Read the model definition and answer for the solid it produces. Units are mm, in the model's axes. A direction names the side the tool comes from. Coordinates: 2 decimals unless noted, no trailing zeros. Write each loop counter-clockwise with the first axis right and the second up, starting at its lowest first coordinate (ties: lowest second). Pieces come first, ordered by that corner, then holes. Notation, with made-up numbers: (9.25, 46) -> (35.25, 46) arc R31 ccw to (35.25, 79) -> close; hole circle Ø9 at (13, 44). An arc over 180 degrees is marked (long way). Answer in a Markdown table with one row per item. Add a question column.
Item 1: Section B-B on y = -35.5 is taken. Write down the section's boundary in (x, z), then the cut area to 3 significant figures.
Item 2: Section A-A on z = 48 is taken. Write down the section's boundary in (x, y).
Item 3: Straight lines are drawn through the part: line 1 (Z direction, x = 10, y = -40); line 2 (Y direction, x = 18, z = 34.5). For each, find the intervals that lie inside material, in ascending order. Write a range as from..to.
Item 4: Section D-D on y = -10 is taken. Write down the section's boundary in (x, z), then the cut area to 3 significant figures.
Item 5: Given pin 1 Ø1.6 at (y, z) = (7.5, 41.5) entering from +X; pin 2 Ø3 at (x, y) = (12.5, -49.5) entering from +Z; pin 3 Ø20 at (y, z) = (-50, 18.5) entering from +X; pin 4 Ø1 at (y, z) = (-24.5, 22.5) entering from -X, each flat-ended and moving along its own axis, determine where each tip first touches the part or whether it passes through.
Item 6: Section C-C on z = 34 is taken. Write down the section's boundary in (x, y).
Item 7: For a pull along Y with two mould halves and no side action, classify faces 5 (the face through (8, -45, 44.852)), 6 (the face through (29, 12.038, 43)), 7 (the face through (29, 3, 40.223)), 8 (the face through (23, -33.682, 35)) as +Y half, -Y half, draft (parallel to the pull), parting line (faces both ways), or undercut.
Item 8: Which of the six approach directions +Z, -Z, +X, -X, +Y, -Y give full straight-line access (tool end or side, diameter ignored) to faces 1 (the face through (25, -31.142, 31)), 2 (the face through (8, -45, 29.717)), 3 (the face through (3.918, -33.197, 34.806)), 4 (the face through (2.54, -46, 49))?
```python
from build123d import *

# Parameters (mm, degrees)
F0_W        = 28.7528
F0_H        = 19.3099416792
F1_DEPTH    = 38.354
F2_DEPTH    = 25.146
F3_R        = 20.8491483247
F5_DEPTH    = 29.972
F6_T        = 2.54
F6_T3_DEPTH = 33.8328
F8_W        = 5.5572818965
F8_H        = 5.2297823131
F9_DEPTH    = 17.78
F9_FACE_W   = 5.5572818965
F9_FACE_H   = 5.2297823131
F7_W        = 38.354
F7_H        = 44.4559416792
F7_R        = 5.5881190885
F10_DEPTH   = 25.4


# Not quite as in the source:
# - a shell that OpenCascade refuses in one call is made with other operations: the cavity is built on its own and cut out


with BuildPart() as f1:
    # F0 (on Right) → F1 (new body)
    with BuildSketch(Plane.YZ):
        with Locations((-45.5179288597, 21.1969297379)):
            Rectangle(F0_W, F0_H)
    extrude(amount=F1_DEPTH)

    # F2 (add): a face of the model
    f2_faces = [f1.faces().sort_by_distance(p)[0] for p in [
        (19.177, -45.5179288597, 30.8519005775),
    ]]
    extrude(f2_faces, amount=F2_DEPTH)

    # F3
    f3_edges = [f1.edges().sort_by_distance(p)[0] for p in [
        (38.354, -59.894329, 33.76993),
    ]]
    fillet(f3_edges, radius=F3_R)

    # F4 (on face) → F5 (cut)
    with BuildSketch(Plane.XZ.offset(59.8943288597)):
        Polygon((5.3893399472, 32.2574861348), (11.1945441877, 32.2574861348), (14.0971463079, 37.2849404812), (11.1945441877, 42.3123948276), (5.3893399472, 42.3123948276), (2.486737827, 37.2849404812), align=None)
    extrude(amount=-F5_DEPTH, mode=Mode.SUBTRACT)

    # F6: shell of thickness 2.54, made by hand


with BuildPart() as f6_core1:
    # F6_t2: copy of F1
    add(f1.part)

    # the walls: a layer under each face that stays
    f6_faces = [f6_core1.faces().sort_by_distance(p)[0] for p in [
        (14.5873763961, -59.8943288597, 48.5885769643),
        (19.177, -45.5179288597, 11.5419588983),
        (32.2474258377, -53.7877546974, 33.7699297379),
        (0, -45.5179288597, 33.7699297379),
        (3.9380388871, -45.5179288597, 39.7986676544),
        (8.2919420674, -45.5179288597, 42.3123948276),
        (12.6458452478, -45.5179288597, 39.7986676544),
        (12.6458452478, -45.5179288597, 34.771213308),
        (8.2919420674, -45.5179288597, 32.2574861348),
        (3.9380388871, -45.5179288597, 34.771213308),
        (38.354, -35.0933546974, 33.7699297379),
        (19.177, -31.1415288597, 33.7699297379),
    ]]
    thicken(f6_faces, amount=-F6_T, mode=Mode.SUBTRACT)

    # F6_s4 → F6_t3 (cut)
    with BuildSketch(Plane.XZ.offset(28.6015288597)):
        Polygon((2.5307319175, 37.2849404812), (0.2870333013, 38.5549404812), (-0.4462015405, 37.2849404812), (0.2870333013, 36.0149404812), align=None)
        Polygon((5.4113369925, 42.2742948276), (3.1896354216, 43.5823948276), (3.9228702635, 44.8523948276), (5.3893399472, 44.8523948276), align=None)
        Polygon((11.1725471424, 42.2742948276), (11.1945441877, 44.8523948276), (12.6610138714, 44.8523948276), (13.3942487133, 43.5823948276), align=None)
        Polygon((14.0531522174, 37.2849404812), (16.2968508335, 38.5549404812), (17.0300856754, 37.2849404812), (16.2968508335, 36.0149404812), align=None)
        Polygon((11.1725471424, 32.2955861348), (13.3942487133, 30.9874861348), (12.6610138714, 29.7174861348), (11.1945441877, 29.7174861348), align=None)
        Polygon((5.4113369925, 32.2955861348), (5.3893399472, 29.7174861348), (3.9228702635, 29.7174861348), (3.1896354216, 30.9874861348), align=None)
    extrude(amount=F6_T3_DEPTH, mode=Mode.SUBTRACT)


with BuildPart() as f1_1:
    add(f1.part)

    # what is left inside the walls is the cavity
    f6_cavity = [f6_core1.part.solids().sort_by_distance(p)[0] for p in [
        (24.722667, -33.706929, 35.03993),
    ]]
    add(f6_cavity, mode=Mode.SUBTRACT)

    # F8 (on face) → F9 (join)
    with BuildSketch(Plane(origin=(0, -31.1415288597, 0), x_dir=(-1, 0, 0), z_dir=(0, 1, 0))):
        with Locations((-28.6376820877, 42.8374167532)):
            Rectangle(F8_W, F8_H)
    extrude(amount=F9_DEPTH)

    # F9_face (on face) + F7 (on face) → F10 (join)
    with BuildSketch(Plane(origin=(28.6376820877, -13.3615288597, 42.8374167532), x_dir=(-1, 0, 0), z_dir=(0, 1, 0))):
        Rectangle(F9_FACE_W, F9_FACE_H)
    with BuildSketch(Plane(origin=(0, -31.1415288597, 0), x_dir=(-1, 0, 0), z_dir=(0, 1, 0))):
        with Locations((-19.177, 33.7699297379)):
            Rectangle(F7_W, F7_H)
        with Locations((-25.0183418393, 30.7178907096)):
            Circle(F7_R, mode=Mode.SUBTRACT)
        Polygon((-5.3893399472, 42.3123948276), (-2.486737827, 37.2849404812), (-5.3893399472, 32.2574861348), (-11.1945441877, 32.2574861348), (-14.0971463079, 37.2849404812), (-11.1945441877, 42.3123948276), align=None, mode=Mode.SUBTRACT)
    extrude(amount=F10_DEPTH)


solid = f1_1.part
```
Results below:
| question | item | result |
|---|---|---|
| 1 | outline | (0, 11.54) -> (38.35, 11.54) -> (38.35, 56) -> (35.81, 56) -> (35.81, 14.08) -> (2.54, 14.08) -> (2.54, 32.11) -> (3.92, 29.72) -> (12.66, 29.72) -> (17.03, 37.28) -> (12.66, 44.85) -> (3.92, 44.85) -> (2.54, 42.46) -> (2.54, 56) -> (0, 56) -> close; hole (2.49, 37.28) -> (5.39, 32.26) -> (11.19, 32.26) -> (14.1, 37.28) -> (11.19, 42.31) -> (5.39, 42.31) -> close |
| 1 | area | 406 mm2 |
| 2 | outline | (0, -59.89) -> (17.5, -59.89) arc R20.85 ccw to (38.35, -39.05) -> (38.35, -5.74) -> (0, -5.74) -> close; hole (2.54, -57.35) -> (17.5, -57.35) arc R18.31 ccw to (35.81, -39.05) -> (35.81, -33.68) -> (2.54, -33.68) -> close |
| 3 | line 1 | z = 11.54..14.08, 29.72..32.26, 42.31..44.85 |
| 3 | line 2 | y = -59.89..-57.35, -33.68..-5.74 |
| 4 | outline | (0, 11.54) -> (38.35, 11.54) -> (38.35, 56) -> (0, 56) -> close; hole (2.49, 37.28) -> (5.39, 32.26) -> (11.19, 32.26) -> (14.1, 37.28) -> (11.19, 42.31) -> (5.39, 42.31) -> close; hole circle Ø11.18 at (25.02, 30.72) |
| 4 | area | 1,520 mm2 |
| 5 | pin 1 | stops at x = 31.42 |
| 5 | pin 2 | stops at z = 44.85 |
| 5 | pin 3 | stops at x = 38.33 |
| 5 | pin 4 | stops at x = 0 |
| 6 | outline | (0, -59.89) -> (4.38, -59.89) -> (4.38, -5.74) -> (0, -5.74) -> close; (12.2, -59.89) -> (17.5, -59.89) arc R20.85 ccw to (38.35, -39.05) -> (38.35, -5.74) -> (29.54, -5.74) -> (29.54, -31.14) -> (20.5, -31.14) -> (20.5, -5.74) -> (12.2, -5.74) -> close; hole (15.13, -57.35) -> (17.5, -57.35) arc R18.31 ccw to (35.81, -39.05) -> (35.81, -33.68) -> (15.13, -33.68) -> close |
| 7 | face 5 | undercut |
| 7 | face 6 | +Y half |
| 7 | face 7 | draft |
| 7 | face 8 | undercut |
| 8 | face 1 | +Y |
| 8 | face 2 | none |
| 8 | face 3 | +Y, -Y |
| 8 | face 4 | +Z |
